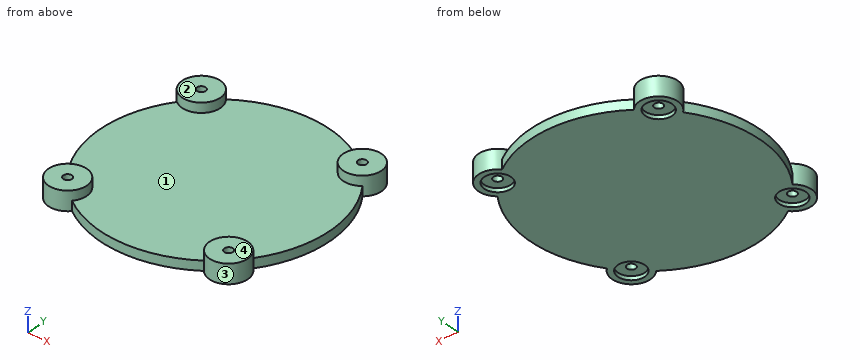
Solid Edge part; units mm, degrees
sketch "Sketch1" plane through (0, 0, 0) normal (0, 0, 1) x (1, 0, 0)
  circle A0 centre (0.8667, -4.8625) radius 60
extrude "Protrusion1" add sketch "Sketch1" along normal blind 5
sketch "Sketch2" plane through (0, 0, 0) normal (0, 0, 1) x (1, 0, 0)
  circle A0 centre (-41.5597, -47.289) radius 10
  circle A1 centre (-41.5597, 37.5639) radius 10
  circle A2 centre (43.2931, -47.289) radius 10
  circle A3 centre (43.2931, 37.5639) radius 10
extrude "ExtrudedProtrusion_2" add sketch "Sketch2" along normal blind 10
sketch "Sketch3" plane through (-41.5597, -47.289, 10) normal (0, 0, 1) x (1, 0, 0)
  circle A0 centre (0, 0) radius 2.25
  circle A1 centre (0, 84.8528) radius 2.25
  circle A2 centre (84.8528, 0) radius 2.25
  circle A3 centre (84.8528, 84.8528) radius 2.25
extrude "Cutout1" cut sketch "Sketch3" against normal up to next
sketch "Sketch4" plane through (0.8667, -4.8625, 0) normal (0, 0, -1) x (1, 0, 0)
  circle A0 centre (-42.4264, -42.4264) radius 7
  circle A1 centre (42.4264, -42.4264) radius 7
  circle A2 centre (42.4264, 42.4264) radius 7
  circle A3 centre (-42.4264, 42.4264) radius 7
extrude "ExtrudedCutout_2" cut sketch "Sketch4" against normal blind 2
The model under review builds one solid part; all positions refer to its coordinate system, in mm. Face numbers are marked on the shaded views. A direction names the side the tool comes from. Round coordinates to 2 decimals unless told otherwise and drop trailing zeros. Order: outer loops, then holes, each group sorted by start corner. A loop starts at its lowest first (then second) coordinate and runs counter-clockwise, first axis right, second up. Notation, with made-up numbers: (3.25, 33) -> (13.25, 33) arc R24 ccw to (13.25, 65) -> close; hole circle Ø9 at (4.25, 18.5). An arc over 180 degrees is marked (long way). Use CSV: the item, a comma, the result in double quotes. Start each with the question number.
(1) Mouldability with a two-part tool opening along Y and no side actions: class the marked faces 1 and 2 as pulls with the +Y half, pulls with the -Y half, needs draft (parallel to the pull), parting line crosses it, or undercut.
(2) Consider section B-B on x = -36.5. Write out the cut boundary in (y, z), and give its area (3 significant figures).
(3) Consider section C-C on y = 6. Write out the cut boundary in (x, z).
(4) Wall thickness on probe 1 along Y at (x, z) = (43, 6.5); probe 2 along X at (y, z) = (-47, 3.25); probe 3 along Y at (x, z) = (-40, 5.5): over which ranges is each line inside the solid? List them lowest first. Write a range as from..to.
(5) Insertion check: pin 1 (11 mm diameter, centred on x = -41, y = -48.5, fed in from -Z); pin 2 (4 mm diameter, centred on x = -46.5, z = 5, fed in from -Y); pin 3 (10 mm diameter, centred on x = -41.5, y = -1.5, fed in from +Z). Each pin has a flat end and moves straight along its axis. Give the tip position at first contact, or say it passes through.
(6) Consider section D-D on y = -35.5. Write out the cut boundary in (x, z).
(7) Consider section A-A on z = 8.5. Write out the cut boundary in (x, y).
(8) Tool access review of the marked faces 3 and 4: name each direction out of +Z, -Z, +X, -X, +Y, -Y from which nothing blocks a thin tool from reaching the whole face with its end or side.
Responses:
1,face 1,"undercut"
1,face 2,"needs draft"
2,outline,"(-55.91, 0) -> (-52.13, 0) -> (-52.13, 2) -> (-42.45, 2) -> (-42.45, 0) -> (32.73, 0) -> (32.73, 2) -> (42.4, 2) -> (42.4, 0) -> (46.19, 0) -> (46.19, 10) -> (28.94, 10) -> (28.94, 5) -> (-38.66, 5) -> (-38.66, 10) -> (-55.91, 10) -> close"
2,area,"644 mm²"
3,outline,"(-58.14, 0) -> (59.88, 0) -> (59.88, 5) -> (-58.14, 5) -> close"
4,probe 1,"-57.28..-49.52, -45.06..-37.29, 27.57..35.33, 39.79..47.56"
4,probe 2,"-51.56..-43.79, -39.33..41.06, 45.52..53.29"
4,probe 3,"-57.17..-48.91, -45.67..-37.41, 27.69..35.94, 39.19..47.44"
5,pin 1,"z = 2"
5,pin 2,"y = -56.85"
5,pin 3,"z = 5"
6,outline,"(-50.72, 0) -> (52.45, 0) -> (52.45, 5) -> (-50.72, 5) -> close"
7,outline,"circle Ø20 at (-41.56, -47.29); circle Ø20 at (-41.56, 37.56); circle Ø20 at (43.29, -47.29); circle Ø20 at (43.29, 37.56); hole circle Ø4.5 at (-41.56, -47.29); hole circle Ø4.5 at (-41.56, 37.56); hole circle Ø4.5 at (43.29, -47.29); hole circle Ø4.5 at (43.29, 37.56)"
8,face 3,"+Z"
8,face 4,"+Z, +X, -X, +Y, -Y"
